Here's how the part is built. I have some questions about the finished solid (model axes, mm). Face numbers are marked on the shaded views. A direction names the side the tool comes from. Coordinates: 2 decimals unless noted, no trailing zeros. Order: outer loops, then holes, each group sorted by start corner. A loop starts at its lowest first (then second) coordinate and runs counter-clockwise, first axis right, second up. Notation, with made-up numbers: (-18.75, 87) - (-4.75, 87) arc R25 ccw to (-4.75, 117) - close; hole circle Ø2 at (-40, 70). An arc over 180 degrees is marked (long way). Answer in a Markdown table with one row per item. Add a question column.
Item 1: I want a section at A-A (x = 197). Please give me the cut outline in (y, z).
Item 2: On a 3-axis mill with a long thin cutter (end or side, diameter ignored), from which of +Z, -Z, +X, -X, +Y, -Y can I reach the whole of each face in a straight line? I mean the marked faces 5 and 6. Say none if no direction works.
Item 3: Will these pins go through, and if not, where does the flat tip stop? pin 1 Ø10 at (y, z) = (10.5, -32.5) entering from -X; pin 2 Ø20.5 at (x, y) = (27, -1) entering from -Z; pin 3 Ø6 at (y, z) = (-14.5, -82) entering from +X.
Item 4: I want a section at B-B (z = 112). Please give me the cut outline in (x, y), plus the area to 3 significant figures.
Item 5: Thinking about a two-plate mould opening in Z: for the marked faces 1, 2, 3 and 4, which applies, +Z half, -Z half, draft (parallel to the pull), parting line (faces both ways), or undercut?
Item 6: If I drill on line 1 along X through (y, z) = (7, 112); line 2 along X through (y, z) = (7.5, 37); line 3 along Z through (x, y) = (-87.5, 0), over which ranges is the centre line in solid material (lowest first)? Write a range as from..to.
Item 7: I want a section at D-D (y = 15). Please give me the cut outline in (x, z).
Item 8: I want a section at C-C (x = -12). Please give me the cut outline in (y, z).
```python
from build123d import *

# Parameters (mm, degrees)
SKETCH1_W           = 416
SKETCH1_H           = 246
BOSS_EXTRUDE1_DEPTH = 20.5
SKETCH2_W           = 372
SKETCH2_H           = 202
CUT_EXTRUDE1_DEPTH  = 30
SKETCH3_R           = 24
BOSS_EXTRUDE2_DEPTH = 20.5
SKETCH4_R           = 17.5
CUT_EXTRUDE2_DEPTH  = 30


with BuildPart() as part:
    # Sketch1 → Boss-Extrude1 (new, symmetric)
    with BuildSketch(Plane(origin=(0, 0, 0), x_dir=(1, 0, 0), z_dir=(0, 1, 0))):
        Rectangle(SKETCH1_W, SKETCH1_H)
    extrude(amount=BOSS_EXTRUDE1_DEPTH, both=True)

    # Sketch2 → Cut-Extrude1 (cut, symmetric)
    with BuildSketch(Plane(origin=(0, 0, 0), x_dir=(1, 0, 0), z_dir=(0, 1, 0))):
        Rectangle(SKETCH2_W, SKETCH2_H)
    extrude(amount=CUT_EXTRUDE1_DEPTH, both=True, mode=Mode.SUBTRACT)

    # Sketch3 → Boss-Extrude2 (add, symmetric)
    with BuildSketch(Plane(origin=(0, 0, 0), x_dir=(1, 0, 0), z_dir=(0, 1, 0))):
        with Locations((-197, -112)):
            Circle(SKETCH3_R)
        with Locations((-197, 112)):
            Circle(SKETCH3_R)
        with Locations((197, -112)):
            Circle(SKETCH3_R)
        with Locations((197, 112)):
            Circle(SKETCH3_R)
    extrude(amount=BOSS_EXTRUDE2_DEPTH, both=True)

    # Sketch4 → Cut-Extrude2 (cut, symmetric)
    with BuildSketch(Plane(origin=(0, 0, 0), x_dir=(1, 0, 0), z_dir=(0, 1, 0))):
        with Locations(Location((-197, -112, 0), (0, 0, 270))):
            Circle(SKETCH4_R)
        with Locations(Location((-197, 112, 0), (0, 0, 270))):
            Circle(SKETCH4_R)
        with Locations(Location((197, -112, 0), (0, 0, 270))):
            Circle(SKETCH4_R)
        with Locations(Location((197, 112, 0), (0, 0, 270))):
            Circle(SKETCH4_R)
    extrude(amount=CUT_EXTRUDE2_DEPTH, both=True, mode=Mode.SUBTRACT)


solid = part.part
```
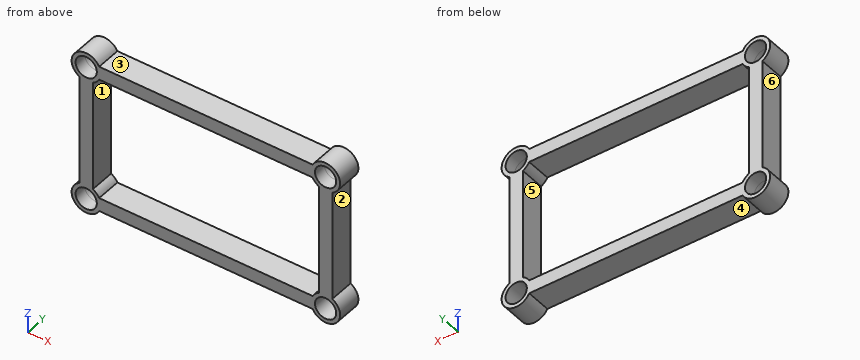
Values follow:
| question | item | result |
|---|---|---|
| 1 | outline | (-20.5, -136) - (20.5, -136) - (20.5, -129.5) - (-20.5, -129.5) - close; (-20.5, -94.5) - (20.5, -94.5) - (20.5, 94.5) - (-20.5, 94.5) - close; (-20.5, 129.5) - (20.5, 129.5) - (20.5, 136) - (-20.5, 136) - close |
| 2 | face 5 | +Y, -Y |
| 2 | face 6 | -X, +Y, -Y |
| 3 | pin 1 | stops at x = -208 |
| 3 | pin 2 | stops at z = -123 |
| 3 | pin 3 | stops at x = 208 |
| 4 | outline | (-221, -20.5) - (-214.5, -20.5) - (-214.5, 20.5) - (-221, 20.5) - close; (-179.5, -20.5) - (179.5, -20.5) - (179.5, 20.5) - (-179.5, 20.5) - close; (214.5, -20.5) - (221, -20.5) - (221, 20.5) - (214.5, 20.5) - close |
| 4 | area | 15,300 mm^2 |
| 5 | face 1 | undercut |
| 5 | face 2 | undercut |
| 5 | face 3 | +Z half |
| 5 | face 4 | -Z half |
| 6 | line 1 | x = -221..-214.5, -179.5..179.5, 214.5..221 |
| 6 | line 2 | x = -208..-186, 186..208 |
| 6 | line 3 | z = -123..-101, 101..123 |
| 7 | outline | (-208, -90.67) arc R24 ccw (long way) to (-175.67, -123) - (175.67, -123) arc R24 ccw (long way) to (208, -90.67) - (208, 90.67) arc R24 ccw (long way) to (175.67, 123) - (-175.67, 123) arc R24 ccw (long way) to (-208, 90.67) - close; hole circle Ø35 at (-197, -112); hole circle Ø35 at (-197, 112); hole (-186, -90.67) arc R24 cw to (-175.67, -101) - (175.67, -101) arc R24 cw to (186, -90.67) - (186, 90.67) arc R24 cw to (175.67, 101) - (-175.67, 101) arc R24 cw to (-186, 90.67) - close; hole circle Ø35 at (197, -112); hole circle Ø35 at (197, 112) |
| 8 | outline | (-20.5, -123) - (20.5, -123) - (20.5, -101) - (-20.5, -101) - close; (-20.5, 101) - (20.5, 101) - (20.5, 123) - (-20.5, 123) - close |
